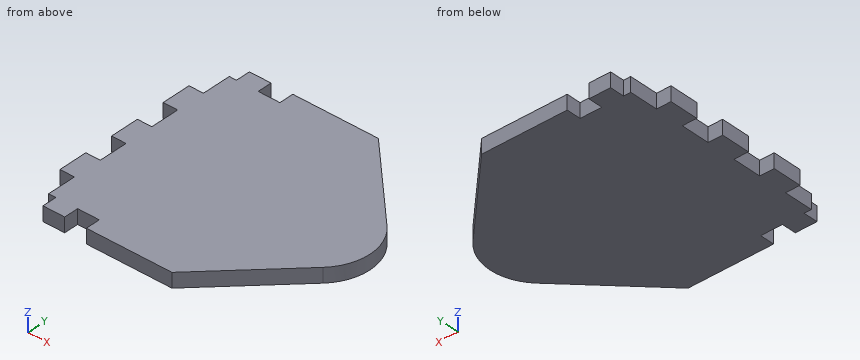
from build123d import *

# Parameters (mm, degrees)
BOSS_EXTRUDE1_DEPTH = 6.35
CAVITY2_START       = -19.05
CAVITY2_OUTLINE_W   = 19.05
CAVITY2_OUTLINE_H   = 6.35
CAVITY2_OUTLINE_W_2 = 12.7
CAVITY2_DEPTH       = 6.350000002
CAVITY2_2_OUTLINE_W = 6.35
CAVITY2_2_OUTLINE_H = 6.35
CAVITY2_2_DEPTH     = 9.525
CAVITY2_START_2     = -12.699999998
CAVITY2_3_OUTLINE_W = 6.35
CAVITY2_3_OUTLINE_H = 6.35
CAVITY2_3_DEPTH     = 3.174999998


# Read off the part's stored shape, not the designer's step: Cavity2
with BuildPart() as part:
    # Sketch1 → Boss-Extrude1 (new body)
    with BuildSketch(Plane.XY):
        with BuildLine():
            Line((-19.05, -37.547541155), (47.072541155, -37.547541155))
            Line((47.072541155, -37.547541155), (82.157092943, -72.632092943))
            ThreePointArc((82.157092943, -72.632092943), (88.666644731, -88.347541155), (82.157092943, -104.062989367))
            Line((82.157092943, -104.062989367), (47.072541155, -139.147541155))
            Line((47.072541155, -139.147541155), (-19.05, -139.147541155))
            Line((-19.05, -139.147541155), (-19.05, -37.547541155))
        make_face()
    extrude(amount=-BOSS_EXTRUDE1_DEPTH)

    # Cavity2 outline → Cavity2 (cut)
    with BuildSketch(Plane.YZ.offset(CAVITY2_START)):
        with Locations((-129.622541155, -3.175)):
            Rectangle(CAVITY2_OUTLINE_W, CAVITY2_OUTLINE_H)
        with Locations((-101.047541155, -3.175)):
            Rectangle(CAVITY2_OUTLINE_W_2, CAVITY2_OUTLINE_H)
        with Locations((-75.647541155, -3.175)):
            Rectangle(CAVITY2_OUTLINE_W_2, CAVITY2_OUTLINE_H)
        with Locations((-47.072541155, -3.175)):
            Rectangle(CAVITY2_OUTLINE_W, CAVITY2_OUTLINE_H)
    extrude(amount=CAVITY2_DEPTH, mode=Mode.SUBTRACT)

    # Cavity2 2 outline → Cavity2 2 (cut)
    with BuildSketch(Plane.YZ):
        with Locations((-135.972541155, -3.175)):
            Rectangle(CAVITY2_2_OUTLINE_W, CAVITY2_2_OUTLINE_H)
        with Locations((-40.722541155, -3.175)):
            Rectangle(CAVITY2_2_OUTLINE_W, CAVITY2_2_OUTLINE_H)
    extrude(amount=CAVITY2_2_DEPTH, mode=Mode.SUBTRACT)

    # Cavity2 3 outline → Cavity2 3 (cut)
    with BuildSketch(Plane.YZ.offset(CAVITY2_START_2)):
        with Locations((-135.972541155, -3.175)):
            Rectangle(CAVITY2_3_OUTLINE_W, CAVITY2_3_OUTLINE_H)
        with Locations((-40.722541155, -3.175)):
            Rectangle(CAVITY2_3_OUTLINE_W, CAVITY2_3_OUTLINE_H)
    extrude(amount=CAVITY2_3_DEPTH, mode=Mode.SUBTRACT)


solid = part.part
Geometry check sheet. Reference: the model listing, model coordinates, mm. Coordinates: 2 decimals unless noted, no trailing zeros. Order: outer loops, then holes, each group sorted by start corner. A loop starts at its lowest first (then second) coordinate and runs counter-clockwise, first axis right, second up. Notation, with made-up numbers: (29.25, -22) - (86.25, -22) arc R12 ccw to (86.25, -6) - close; hole circle Ø9 at (11, 64.25). An arc over 180 degrees is marked (long way). One line per item, written item: value.
(1) Depth check by flat-ended pin: pin 1 Ø1.9 at (y, z) = (-137.5, -2.5) entering from +X; pin 2 Ø1.9 at (y, z) = (-41, -2) entering from +X (3 decimals); pin 3 Ø1.9 at (x, z) = (6, -3) entering from -Y. Enter the tip coordinate at first touch or a pass-through.
Data:
pin 1: stops at x = 49.67
pin 2: stops at x = 51.475
pin 3: stops at y = -132.8
(2) Thickness scan on probe 1 along Y at (x, z) = (5, -2); probe 2 along X at (y, z) = (-43, -3) (3 decimals); probe 3 along X at (y, z) = (-134.5, -3.75) (3 decimals). Record the ranges inside material, lowest first. Write a range as from..to.
Data:
probe 1: y = -132.8..-43.9
probe 2: x = -9.525..0, 9.525..52.525
probe 3: x = -9.525..0, 9.525..51.72
(3) Sectioned sample at C-C (y = -77.5). Enter the section's corners in (x, z), and give its area (3 significant figures).
Data:
outline: (-12.7, -6.35) - (85.84, -6.35) - (85.84, 0) - (-12.7, 0) - close
area: 626 mm^2
(4) Sectioned sample at B-B (x = 4.5). Enter the section's corners in (y, z).
Data:
outline: (-132.8, -6.35) - (-43.9, -6.35) - (-43.9, 0) - (-132.8, 0) - close
